The model under review builds one solid part; all positions refer to its coordinate system, in mm. A direction names the side the tool comes from. Give positions to 0.01 mm unless a question says otherwise; leave off trailing zeros. Order: outer loops, then holes, each group sorted by start corner. A loop starts at its lowest first (then second) coordinate and runs counter-clockwise, first axis right, second up.
```python
from build123d import *

# Parameters (mm, degrees)
SKETCH1_W           = 177.8
SKETCH1_H           = 127
SKETCH1_R           = 5.588
SKETCH1_R_2         = 1.4605
SKETCH1_W_2         = 28.956
SKETCH1_H_2         = 59.69
BOSS_EXTRUDE1_DEPTH = 12.7
SKETCH3_W           = 8.128
SKETCH3_H           = 35.052
CUT_EXTRUDE3_DEPTH  = 13.7
SKETCH2_W           = 44.45
SKETCH2_H           = 79.4004
CUT_EXTRUDE4_DEPTH  = 5.08


with BuildPart() as part:
    # Sketch1 → Boss-Extrude1 (new body)
    with BuildSketch(Plane(origin=(0, 0, 0), x_dir=(1, 0, 0), z_dir=(0, 1, 0))):
        Rectangle(SKETCH1_W, SKETCH1_H)
        with Locations((-63.5, 0)):
            Circle(SKETCH1_R, mode=Mode.SUBTRACT)
        with Locations((63.5, 0)):
            Circle(SKETCH1_R, mode=Mode.SUBTRACT)
        with Locations((-5.667565537, -42.871775783)):
            Circle(SKETCH1_R_2, mode=Mode.SUBTRACT)
        with Locations((10.207434463, -42.871775783)):
            Circle(SKETCH1_R_2, mode=Mode.SUBTRACT)
        with Locations((-5.667565537, 25.149424217)):
            Circle(SKETCH1_R_2, mode=Mode.SUBTRACT)
        with Locations((10.207434463, 25.149424217)):
            Circle(SKETCH1_R_2, mode=Mode.SUBTRACT)
        with Locations((2.269934463, -8.661150783)):
            Rectangle(SKETCH1_W_2, SKETCH1_H_2, mode=Mode.SUBTRACT)
    extrude(amount=BOSS_EXTRUDE1_DEPTH)

    # Sketch3 → Cut-Extrude3 (cut, through all)
    with BuildSketch(Plane(origin=(0, 0, 0), x_dir=(1, 0, 0), z_dir=(0, 1, 0))):
        with Locations((-16.19114245, -24.615525783)):
            Rectangle(SKETCH3_W, SKETCH3_H)
        with Locations((20.731011375, -24.615525783)):
            Rectangle(SKETCH3_W, SKETCH3_H)
    extrude(amount=CUT_EXTRUDE3_DEPTH, mode=Mode.SUBTRACT)

    # Sketch2 → Cut-Extrude4 (cut)
    with BuildSketch(Plane(origin=(0, 12.7, 0), x_dir=(1, 0, 0), z_dir=(0, 1, 0))):
        with Locations((2.269934463, -8.737350783)):
            Rectangle(SKETCH2_W, SKETCH2_H)
    extrude(amount=-CUT_EXTRUDE4_DEPTH, mode=Mode.SUBTRACT)


solid = part.part
```
Item 1: Take a section at A-A (z = 0). Give the boundary of the cut face in (x, y), and give its area (3 significant figures).
Values found:
outline: (-88.9, 0) - (-69.09, 0) - (-69.09, 12.7) - (-88.9, 12.7) - close; (-57.91, 0) - (-12.21, 0) - (-12.21, 7.62) - (-19.96, 7.62) - (-19.96, 12.7) - (-57.91, 12.7) - close; (16.75, 0) - (57.91, 0) - (57.91, 12.7) - (24.49, 12.7) - (24.49, 7.62) - (16.75, 7.62) - close; (69.09, 0) - (88.9, 0) - (88.9, 12.7) - (69.09, 12.7) - close
area: 1,530 mm2
Item 2: Take a section at D-D (y = 4.75). Give the boundary of the cut face in (x, z), and give its area (3 significant figures).
Values found:
outline: (-88.9, -63.5) - (88.9, -63.5) - (88.9, 63.5) - (-88.9, 63.5) - close; hole circle Ø11.18 at (-63.5, 0); hole (-20.26, 7.09) - (-12.21, 7.09) - (-12.21, -21.18) - (16.75, -21.18) - (16.75, 7.09) - (24.8, 7.09) - (24.8, 42.14) - (16.67, 42.14) - (16.67, 38.51) - (-12.13, 38.51) - (-12.13, 42.14) - (-20.26, 42.14) - close; hole circle Ø2.92 at (-5.67, -25.15); hole circle Ø2.92 at (-5.67, 42.87); hole circle Ø2.92 at (10.21, -25.15); hole circle Ø2.92 at (10.21, 42.87); hole circle Ø11.18 at (63.5, 0)
area: 20,100 mm2
Item 3: Clearance check with a flat-ended pin moving along its axis: pin 1 Ø19 at (x, z) = (10, -19.5) entering from +Y. State where the tip first meets the part, or that it passes through.
Values found:
pin 1: stops at y = 7.62
Item 4: Take a section at C-C (z = 16). Give the boundary of the cut face in (x, y), and give its area (3 significant figures).
Values found:
outline: (-88.9, 0) - (-20.26, 0) - (-20.26, 12.7) - (-88.9, 12.7) - close; (24.8, 0) - (88.9, 0) - (88.9, 12.7) - (24.8, 12.7) - close
area: 1,690 mm2
Item 5: For faces 4 (the flat face through (-21, 0, -1)), 5 (the flat face through (-19.955, 10, -12)), 6 (the flat face through (-16, 3, 7.09)), list the 3-axis set-ups (+Z, -Z, +X, -X, +Y, -Y) from which the entire face can be reached by the end or side of a thin tool; tool diameter is ignored.
Values found:
face 4: +Z, -Z, +X, -X, -Y
face 5: +Y
face 6: +Y, -Y
Item 6: Take a section at B-B (x = -63.5). Give the boundary of the cut face in (y, z), and give its area (3 significant figures).
Values found:
outline: (0, -63.5) - (12.7, -63.5) - (12.7, -5.59) - (0, -5.59) - close; (0, 5.59) - (12.7, 5.59) - (12.7, 63.5) - (0, 63.5) - close
area: 1,470 mm2
Item 7: For line 1 (Z direction, x = -7.5, y = 8); line 2 (X direction, y = 5.25, z = 21); line 3 (Z direction, x = 15.5, y = 0.5), list the stretches that pass through material, from the lowest coordinate up.
Values found:
line 1: z = -63.5 to -30.96, 48.44 to 63.5
line 2: x = -88.9 to -20.26, 24.8 to 88.9
line 3: z = -63.5 to -21.18, 38.51 to 63.5
Item 8: Draft analysis for pull direction X (two halves, no side actions). For faces 1 (the flat face through (24.495, 10, 45)), 2 (the flat face through (-21, 12.7, -1)), 3 (the flat face through (88.9, 6, 1)), state which applies: released by +X, released by -X, zero draft, split by the parting line, or undercut.
Values found:
face 1: undercut
face 2: zero draft
face 3: released by +X
